from build123d import *

# Parameters (mm, degrees)
SKETCH1_R           = 252
BOSS_EXTRUDE1_DEPTH = 50
SKETCH2_R           = 252
SKETCH2_R_2         = 202
BOSS_EXTRUDE2_DEPTH = 1149.92
SKETCH3_R           = 252
BOSS_EXTRUDE3_DEPTH = 50
SKETCH4_R           = 36.45
CUT_EXTRUDE1_DEPTH  = 1300.733821365


with BuildPart() as part:
    # Sketch1 → Boss-Extrude1 (new body)
    with BuildSketch(Plane.XY):
        Circle(SKETCH1_R)
    extrude(amount=BOSS_EXTRUDE1_DEPTH)

    # Sketch2 → Boss-Extrude2 (add)
    with BuildSketch(Plane.XY.offset(50)):
        Circle(SKETCH2_R)
        Circle(SKETCH2_R_2, mode=Mode.SUBTRACT)
    extrude(amount=BOSS_EXTRUDE2_DEPTH)

    # Sketch3 → Boss-Extrude3 (add)
    with BuildSketch(Plane.XY.offset(1199.92)):
        Circle(SKETCH3_R)
    extrude(amount=BOSS_EXTRUDE3_DEPTH)

    # Sketch4 → Cut-Extrude1 (cut, through all)
    with BuildSketch(Plane.XY.offset(1249.92)):
        Circle(SKETCH4_R)
    extrude(amount=-CUT_EXTRUDE1_DEPTH, mode=Mode.SUBTRACT)


solid = part.part
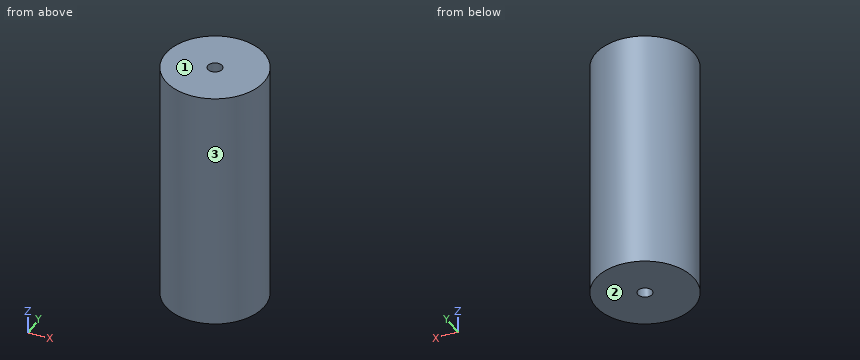
Source: CAD feature listing. Evaluate the final solid. Frame: model axes, mm. Face numbers are marked on the shaded views. Round coordinates to 2 decimals unless told otherwise and drop trailing zeros. Loops run counter-clockwise (first coordinate to the right, second up) from the corner with the lowest first, then second, coordinate; pieces in that order, holes last.
Q1. Section C-C, the plane y = 52.5. Return loops of the section in (x, z).
Q2. Ray query, line 1 (Y direction, x = 0, z = 1226.5); line 2 (Y direction, x = 0, z = 588); line 3 (Z direction, x = 43.5, y = -167.5). Return the intervals inside material, ascending.
Q3. Section A-A, the plane x = 0. Return loops of the section in (y, z), plus the area to 3 significant figures.
Q4. Mould query, pull axis Z, two halves, no side actions, for the marked faces 1, 2 and 3. Classes: pulls with the +Z half, pulls with the -Z half, needs draft (parallel to the pull), parting line crosses it, or undercut.
Q5. First-contact query: P1, Ø8, axis at y = 111, z = 764.5, coming from the -X side; P2, Ø12, axis at x = 138.5, z = 874.5, coming from the -Y side; P3, Ø1.5, axis at x = -123.5, z = 377.5, coming from the -Y side. Flat tips, straight axial feed; report the tip coordinate or a pass-through.
Q6. Section D-D, the plane z = 794. Return loops of the section in (x, y), plus the area to 3 significant figures.
Solutions:
1. outline: (-246.47, 0) - (246.47, 0) - (246.47, 1249.92) - (-246.47, 1249.92) - close; hole (-195.06, 50) - (195.06, 50) - (195.06, 1199.92) - (-195.06, 1199.92) - close
2. line 1: y = -252 to -36.45, 36.45 to 252
2. line 2: y = -252 to -202, 202 to 252
2. line 3: z = 0 to 50, 1199.92 to 1249.92
3. outline: (-252, 0) - (-36.45, 0) - (-36.45, 50) - (-202, 50) - (-202, 1199.92) - (-36.45, 1199.92) - (-36.45, 1249.92) - (-252, 1249.92) - close; (36.45, 0) - (252, 0) - (252, 1249.92) - (36.45, 1249.92) - (36.45, 1199.92) - (202, 1199.92) - (202, 50) - (36.45, 50) - close
3. area: 158,000 mm2
4. face 1: pulls with the +Z half
4. face 2: pulls with the -Z half
4. face 3: needs draft
5. P1: stops at x = -228.16
5. P2: stops at y = -214.35
5. P3: stops at y = -220.08
6. outline: circle Ø504 at (0, 0); hole circle Ø404 at (0, 0)
6. area: 71,300 mm2
